Design review of the part built by this model. Coordinates are the model's own, in mm. A direction names the side the tool comes from. Coordinates: 2 decimals unless noted, no trailing zeros. Write each loop counter-clockwise with the first axis right and the second up, starting at its lowest first coordinate (ties: lowest second). Pieces come first, ordered by that corner, then holes.
Q1. Add section C-C, the plane z = -2.05. Give the boundary of the cut face in (x, y).
Q2. To check wall thickness, follow probe 1 along Y at (x, z) = (-1.7, 0.1); probe 2 along X at (y, z) = (-9.25, 0.5); probe 3 along X at (y, z) = (-5.75, 0). State the ranges of each line that lie inside material, in increasing order.
Q3. Add section D-D, the plane x = 2.3. Give the boundary of the cut face in (y, z), plus the area to 3 significant figures.
Q4. Add section B-B, the plane y = -10.5. Give the boundary of the cut face in (x, z).
Q5. Clearance check with flat-ended pins moving along their axes: pin 1 Ø1 at (x, y) = (-1, -3) entering from -Z; pin 2 Ø2 at (y, z) = (-2.5, 1.5) entering from +X; pin 3 Ø1 at (y, z) = (-9.5, 0.5) entering from -X. State where each tip first meets the part, or that it passes through.
Q6. The part is to be moulded in two halves that separate along Z. For faces 4 (the face through (0, -12, 0)), 5 (the face through (1.108, 2.943, -0.626)), 6 (the face through (0.78, 1.48, 2.48)), 7 (the face through (0, 2, -1.212)), say which applies: +Z half, -Z half, draft (parallel to the pull), parting line (faces both ways), or undercut.
Q7. Add section A-A, the plane x = 0. Give the boundary of the cut face in (y, z).
Q8. Machinability: for faces 1 (the face through (0, 3, 2)), 2 (the face through (-1.05, 2.16, 0.61)), 3 (the face through (0, 0, 2)), which of the approach directions +Z, -Z, +X, -X, +Y, -Y give a long, thin tool a straight path to every point of the face, cutting with its end or side? Answer none if there is none.
from build123d import *

# Parameters (mm, degrees)
SKETCH_1_R          = 2.6
EXTRUDE_1_DEPTH     = 3
CUT_EXTRUDE_1_DEPTH = 1.5
SKETCH_5_R          = 1.5
EXTRUDE_2_DEPTH     = 12
FILLET_1_R          = 0.2


with BuildPart() as part:
    # 草图1 → 凸台-拉伸1 (new body)
    with BuildSketch(Plane(origin=(0, 0, 0), x_dir=(1, 0, 0), z_dir=(0, 1, 0))):
        with Locations(Location((0, 0, 0), (0, 0, 270))):
            Circle(SKETCH_1_R)
    extrude(amount=EXTRUDE_1_DEPTH)

    # 草图2 → 切除-拉伸1 (cut)
    with BuildSketch(Plane(origin=(0, 3, 0), x_dir=(1, 0, 0), z_dir=(0, 1, 0))):
        Polygon((-0.7, 1.212435565), (0.7, 1.212435565), (1.4, 0), (0.7, -1.212435565), (-0.7, -1.212435565), (-1.4, 0), align=None)
    extrude(amount=-CUT_EXTRUDE_1_DEPTH, mode=Mode.SUBTRACT)

    # 草图5 → 凸台-拉伸2 (add)
    with BuildSketch(Plane.XZ):
        with Locations(Location((0, 0, 0), (0, 0, 270))):
            Circle(SKETCH_5_R)
    extrude(amount=EXTRUDE_2_DEPTH)

    # 圆角1
    fillet_1_edges = [part.edges().sort_by_distance(p)[0] for p in [
        (1.05, 3, -0.606217783),
        (1.05, 3, 0.606217783),
        (0, 3, 1.212435565),
        (-1.05, 3, 0.606217783),
        (-1.05, 3, -0.606217783),
        (0, 3, -1.212435565),
    ]]
    fillet(fillet_1_edges, radius=FILLET_1_R)


solid = part.part
Here are the results:
1. outline: (-1.6, 0) - (1.6, 0) - (1.6, 3) - (-1.6, 3) - close
2. probe 1: y = 0 to 3
2. probe 2: x = -1.41 to 1.41
2. probe 3: x = -1.5 to 1.5
3. outline: (0, -1.21) - (3, -1.21) - (3, 1.21) - (0, 1.21) - close
3. area: 7.27 mm2
4. outline: circle Ø3 at (0, 0)
5. pin 1: stops at z = -1.41
5. pin 2: stops at x = 1.41
5. pin 3: stops at x = -1.5
6. face 4: draft
6. face 5: undercut
6. face 6: parting line
6. face 7: undercut
7. outline: (-12, -1.5) - (0, -1.5) - (0, -2.6) - (3, -2.6) - (3, -1.41) arc R0.2 ccw to (2.8, -1.21) - (1.5, -1.21) - (1.5, 1.21) - (2.8, 1.21) arc R0.2 ccw to (3, 1.41) - (3, 2.6) - (0, 2.6) - (0, 1.5) - (-12, 1.5) - close
8. face 1: +Z, -Z, +X, -X, +Y
8. face 2: +Y
8. face 3: -Y
